Model file for the job. Use its own axes, mm. A direction names the side the tool comes from. Coordinates: 2 decimals unless noted, no trailing zeros. Write each loop counter-clockwise with the first axis right and the second up, starting at its lowest first coordinate (ties: lowest second). Pieces come first, ordered by that corner, then holes. Notation, with made-up numbers: (13, -3.5) -> (67, -3.5) arc R29 cw to (67, 32.5) -> close; hole circle Ø7 at (87.25, -27). An arc over 180 degrees is marked (long way). Write item = value, one per line. Start each with the question number.
from build123d import *

# Parameters (mm, degrees)
BOSS_EXTRUDE1_DEPTH = 100
SHELL1_T            = -3
SKETCH2_W           = 56.015644735
SKETCH2_H           = 35
CUT_EXTRUDE1_DEPTH  = 10
SKETCH3_W           = 12.606592538
SKETCH3_H           = 6.980178381
SKETCH3_W_2         = 11.515112664
SKETCH3_H_2         = 6.37986445
CUT_EXTRUDE2_DEPTH  = 10
SKETCH4_W           = 9.169229256
SKETCH4_H           = 5.894504522
CUT_EXTRUDE3_DEPTH  = 10
SKETCH5_W           = 6.776014824
SKETCH5_H           = 5.054240566
CUT_EXTRUDE4_DEPTH  = 10
SKETCH6_W           = 11.990530565
SKETCH6_H           = 7.12730724
CUT_EXTRUDE5_DEPTH  = 10
SKETCH8_W           = 6.563036955
SKETCH8_H           = 5.005706152
CUT_EXTRUDE6_DEPTH  = 10


with BuildPart() as part:
    # Sketch1 → Boss-Extrude1 (new body)
    with BuildSketch(Plane.XY):
        Polygon((-50, 12.5), (-50, 47.5), (29.792740578, 47.5), (50, 12.5), (50, -12.5), (-50, -12.5), align=None)
    extrude(amount=BOSS_EXTRUDE1_DEPTH)

    # Shell1
    shell1_openings = [part.faces().sort_by_distance(p)[0] for p in [
        (0, -12.5, 50),
    ]]
    offset(amount=SHELL1_T, openings=shell1_openings, kind=Kind.INTERSECTION)

    # Sketch2 → Cut-Extrude1 (cut)
    with BuildSketch(Plane.ZY.offset(50)):
        with Locations((51.884685058, 5)):
            Rectangle(SKETCH2_W, SKETCH2_H)
    extrude(amount=-CUT_EXTRUDE1_DEPTH, mode=Mode.SUBTRACT)

    # Sketch3 → Cut-Extrude2 (cut)
    with BuildSketch(Plane(origin=(50, 0, 0), x_dir=(0, 0, -1), z_dir=(1, 0, 0))):
        with Locations((-88.542199405, -9.009910809)):
            Rectangle(SKETCH3_W, SKETCH3_H)
        with Locations((-11.156276384, -9.310067775)):
            Rectangle(SKETCH3_W_2, SKETCH3_H_2)
    extrude(amount=-CUT_EXTRUDE2_DEPTH, mode=Mode.SUBTRACT)

    # Sketch4 → Cut-Extrude3 (cut)
    with BuildSketch(Plane.XY.offset(100)):
        with Locations((18.993403459, 9.968133111)):
            Rectangle(SKETCH4_W, SKETCH4_H)
    extrude(amount=-CUT_EXTRUDE3_DEPTH, mode=Mode.SUBTRACT)

    # Sketch5 → Cut-Extrude4 (cut)
    with BuildSketch(Plane.ZY.offset(50)):
        with Locations((8.609898129, -7.132480119)):
            Rectangle(SKETCH5_W, SKETCH5_H)
        with Locations((91.390101871, -7.132480119)):
            Rectangle(SKETCH5_W, SKETCH5_H)
    extrude(amount=-CUT_EXTRUDE4_DEPTH, mode=Mode.SUBTRACT)

    # Sketch6 → Cut-Extrude5 (cut)
    with BuildSketch(Plane.XY.offset(100)):
        with Locations((39.347077193, -8.93634638)):
            Rectangle(SKETCH6_W, SKETCH6_H)
    extrude(amount=-CUT_EXTRUDE5_DEPTH, mode=Mode.SUBTRACT)

    # Sketch8 → Cut-Extrude6 (cut)
    with BuildSketch(Plane(origin=(50, 0, 0), x_dir=(0, 0, -1), z_dir=(1, 0, 0))):
        with Locations((-32.231091097, -7.194817018)):
            Rectangle(SKETCH8_W, SKETCH8_H)
    extrude(amount=-CUT_EXTRUDE6_DEPTH, mode=Mode.SUBTRACT)


solid = part.part
(1) Saw through at C-C (z = 40). Give the cut face in (x, y).
(2) Drop flat-ended pins along their axis: pin 1 Ø3 at (x, z) = (12.5, 50) entering from -Y; pin 2 Ø2.5 at (x, z) = (-49, 44) entering from -Y; pin 3 Ø5 at (x, z) = (39.5, 50) entering from +Y. Give the stop position or say it passes through.
(3) Saw through at D-D (x = -10.5). Give the cut face in (y, z), then the cut area to 3 significant figures.
(4) 3-axis set-ups, long thin cutter, end or side, ignore diameter. For faces 4 (the face through (-49, -9.66, 91)), 5 (the face through (39, -5.373, 99)), 6 (the face through (-49, 5, 23.877)): which of +Z, -Z, +X, -X, +Y, -Y reach the whole face in a straight line?
(5) Mould opens along Z. For faces 1 (the face through (33.352, -9, 99)), 2 (the face through (1, 18, 100)), 3 (the face through (49, -9, 5.399)) say: released by +Z, released by -Z, zero draft, split by the parting line, or undercut.
(6) Saw through at A-A (z = 93). Give the cut face in (x, y), then the cut area to 3 significant figures.
(7) Saw through at B-B (y = 28). Give the cut face in (x, z).
(8) Drill centre lines: line 1 along Z through (x, y) = (-40.5, 37); line 2 along Y through (x, z) = (28, 34); line 3 along X through (y, z) = (7, 15.5). Where is each one in solid material? Low to high.
Returned:
q1.outline = (-50, 22.5) -> (-47, 22.5) -> (-47, 44.5) -> (28.06, 44.5) -> (47, 11.7) -> (47, -12.5) -> (50, -12.5) -> (50, 12.5) -> (29.79, 47.5) -> (-50, 47.5) -> close
q2.pin_1 = 44.5
q2.pin_2 = 22.5
q2.pin_3 = 35.02
q3.outline = (-12.5, 0) -> (47.5, 0) -> (47.5, 100) -> (-12.5, 100) -> (-12.5, 97) -> (44.5, 97) -> (44.5, 3) -> (-12.5, 3) -> close
q3.area = 642 mm2
q4.face_4 = +X, -X
q4.face_5 = +Z, -Y
q4.face_6 = -X, -Y
q5.face_1 = zero draft
q5.face_2 = released by +Z
q5.face_3 = undercut
q6.outline = (-50, -12.5) -> (-47, -12.5) -> (-47, -9.66) -> (-50, -9.66) -> close; (-50, -4.61) -> (-47, -4.61) -> (-47, 44.5) -> (28.06, 44.5) -> (47, 11.7) -> (47, -5.52) -> (50, -5.52) -> (50, 12.5) -> (29.79, 47.5) -> (-50, 47.5) -> close
q6.area = 563 mm2
q7.outline = (-50, 0) -> (41.05, 0) -> (41.05, 100) -> (-50, 100) -> close; hole (-47, 3) -> (37.59, 3) -> (37.59, 97) -> (-47, 97) -> close
q8.line_1 = 0 to 3, 97 to 100
q8.line_2 = 44.5 to 47.5
q8.line_3 = -50 to -47, 47 to 50
